Here's how the part is built. I have some questions about the finished solid (model axes, mm). Give positions to 0.01 mm unless a question says otherwise; leave off trailing zeros. Order: outer loops, then holes, each group sorted by start corner. A loop starts at its lowest first (then second) coordinate and runs counter-clockwise, first axis right, second up. Notation, with made-up numbers: (42, -32) - (94, -32) arc R14 cw to (94, -10) - close; hole circle Ø8 at (-28.5, 23.25). An arc over 180 degrees is marked (long way). One line per question, with ' | ' between items.
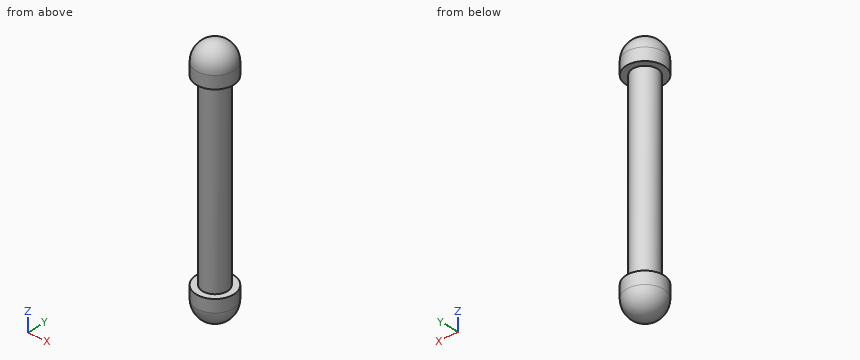
from build123d import *

# Parameters (mm, degrees)
SWEEP1_PROFILE_R     = 2
SKETCH11_R           = 3
BOSS_EXTRUDE1_DEPTH  = 5
FILLET2_R            = 3
FILLET2_OF_MIRROR1_R = 3


with BuildPart() as part:
    # Sweep1: sweep along a path in Sketch1
    with BuildLine(Plane(origin=(0, 0, 0), x_dir=(0, 0, -1), z_dir=(1, 0, 0))) as sweep1_path:
        Line((-14.999999972, 0), (14.999999972, 0))
    # Sweep1 profile (on start of the path) → Sweep1 (sweep)
    with BuildSketch(Plane(origin=(0, 0, 14.999999972), x_dir=(0, -1, 0), z_dir=(0, 0, -1))):
        Circle(SWEEP1_PROFILE_R)
    sweep(path=sweep1_path.line)

    # Sketch11 → Boss-Extrude1 (add)
    with BuildSketch(Plane(origin=(0, 0, -14.999999972), x_dir=(-1, 0, 0), z_dir=(0, 0, -1))):
        with Locations(Location((0, 0, 0), (0, 0, 90))):
            Circle(SKETCH11_R)
    boss_extrude1 = extrude(amount=BOSS_EXTRUDE1_DEPTH)

    # Fillet2
    fillet2_edges = [part.edges().sort_by_distance(p)[0] for p in [
        (0, -3, -19.999999972),
    ]]
    fillet(fillet2_edges, radius=FILLET2_R)

    # Mirror1: Boss-Extrude1 across plane
    add(boss_extrude1.mirror(Plane.XY))

    # Fillet2 of Mirror1
    fillet2_of_mirror1_edges = [part.edges().sort_by_distance(p)[0] for p in [
        (0, -3, 19.999999972),
    ]]
    fillet(fillet2_of_mirror1_edges, radius=FILLET2_OF_MIRROR1_R)


solid = part.part
1) I want a section at C-C (y = 2.5). List the corners of the cut face in (x, z) for me.
Model answer:
outline: (-1.66, -17) arc R1.66 ccw to (1.66, -17) - (1.66, -15) - (-1.66, -15) - close; (-1.66, 15) - (1.66, 15) - (1.66, 17) arc R1.66 ccw to (-1.66, 17) - close
2) I want a section at A-A (y = 0). List the corners of the cut face in (x, z) for me.
Model answer:
outline: (-3, -17) arc R3 ccw to (3, -17) - (3, -15) - (2, -15) - (2, 15) - (3, 15) - (3, 17) arc R3 ccw to (-3, 17) - (-3, 15) - (-2, 15) - (-2, -15) - (-3, -15) - close
3) I'm going to push flat-ended pins straight in: P1, Ø2, axis at y = -1.5, z = -11.5, coming from the -X side; P2, Ø1.8, axis at x = 1.5, y = 0, coming from the +Z side; P3, Ø2, axis at y = -1.5, z = 14.5, coming from the +X side. Where does each tip first touch, or does it pass through?
Model answer:
P1: stops at x = -1.94 | P2: stops at z = 19.94 | P3: stops at x = 2.93
4) Please list where these lines run through material, in increasing order: L1, parallel to Z at x = 2.25, y = 1.4; L2, parallel to Z at x = -2.2, y = -1.15; L3, parallel to X at y = 0.1, z = -13.5.
Model answer:
L1: z = -18.41 to -15, 15 to 18.41 | L2: z = -18.68 to -15, 15 to 18.68 | L3: x = -2 to 2
5) I want a section at D-D (z = 13.5). List the corners of the cut face in (x, y) for me.
Model answer:
outline: circle Ø4 at (0, 0)
